For this review, use the dimensioned drawing (mm, ordinates from the lowest corner) and the shaded views. A direction names the side the tool comes from. Give positions to 0.01 mm unless a question says otherwise; leave off trailing zeros. Write each loop counter-clockwise with the first axis right and the second up, starting at its lowest first coordinate (ties: lowest second). Pieces come first, ordered by that corner, then holes. Notation, with made-up numbers: M 8,-21.5 L 39,-21.5 A33 cw 39,10.5 Z; hole C 46,74.25 d6. An arc over 180 degrees is marked long. One line per item, written item: value. Start each with the question number.
Item 1: Consider section C-C, the plane y = 2.25. Write out the cut boundary in (x, z), and give its area (3 significant figures).
Item 2: To check wall thickness, follow probe 1 along X at (y, z) = (2.75, 12); probe 2 along Z at (x, y) = (12.34, 1.75); probe 3 along Z at (x, y) = (21, 2.5). State the ranges of each line that lie inside material, in increasing order.
Item 3: Consider section B-B, the plane z = 12.34. Write out the cut boundary in (x, y), and give its area (3 significant figures).
Item 4: Mouldability with a two-part tool opening along X and no side actions: class the marked faces 3, 4 and 5 as released by +X, released by -X, zero draft, split by the parting line, or undercut.
Item 5: Consider section A-A, the plane x = 12.34. Write out the cut boundary in (y, z), and give its area (3 significant figures).
Item 6: Tool access review of the marked faces 1 and 2: name each direction out of +Z, -Z, +X, -X, +Y, -Y from which nothing blocks a thin tool from reaching the whole face with its end or side.
Item 7: Consider section D-D, the plane y = 8.25. Write out the cut boundary in (x, z).
Item 8: Clearance check with flat-ended pins moving along their axes: pin 1 Ø11 at (x, z) = (11.5, 12) entering from -Y; pin 2 Ø4 at (y, z) = (6.5, 15) entering from -X; pin 3 Ø2 at (x, z) = (5, 7) entering from -Y. State where each tip first meets the part, or that it passes through.
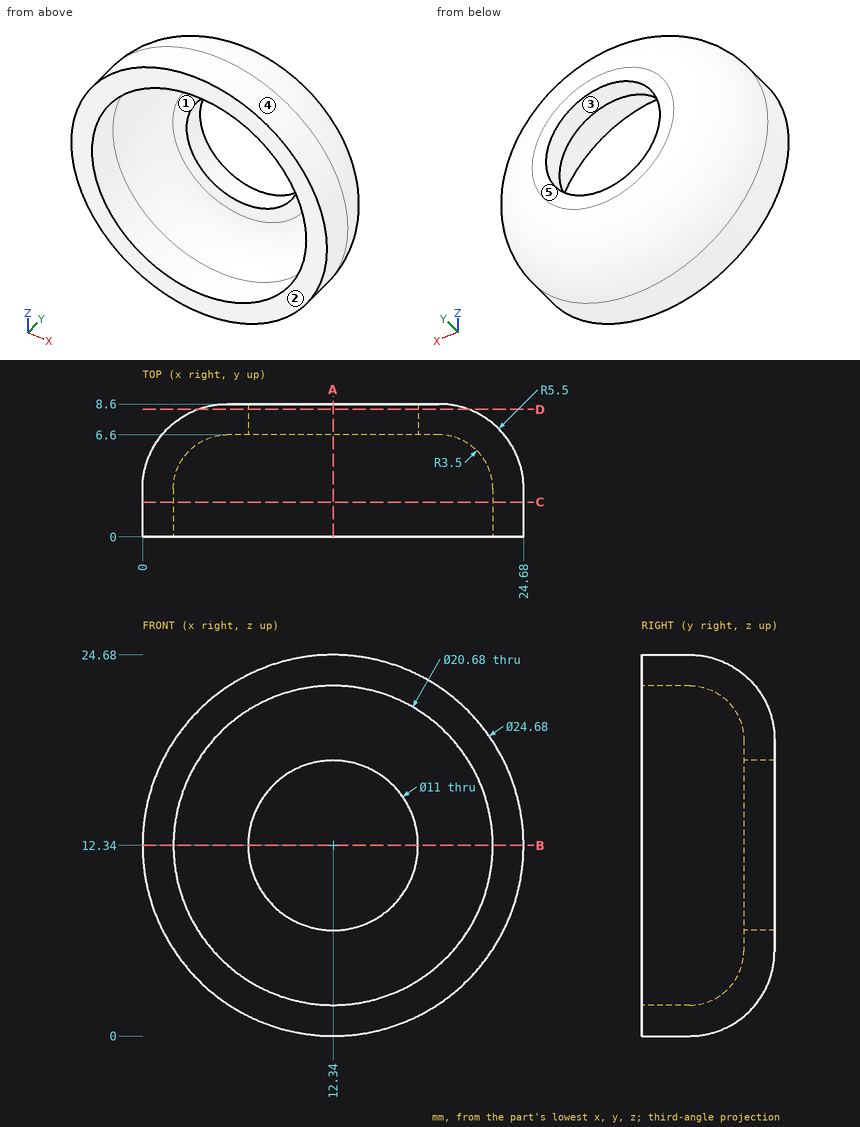
Model answer:
1. outline: C 12.34,12.34 d24.68; hole C 12.34,12.34 d20.68
1. area: 143 mm2
2. probe 1: x = 0 to 2.01, 22.67 to 24.68
2. probe 2: z = 0 to 2, 22.68 to 24.68
2. probe 3: z = 3.55 to 6.69, 17.99 to 21.13
3. outline: M 0,0 L 2,0 L 2,3.1 A3.5 cw 5.5,6.6 L 6.84,6.6 L 6.84,8.6 L 5.5,8.6 A5.5 ccw 0,3.1 Z; M 17.84,6.6 L 19.18,6.6 A3.5 cw 22.68,3.1 L 22.68,0 L 24.68,0 L 24.68,3.1 A5.5 ccw 19.18,8.6 L 17.84,8.6 Z
3. area: 46.0 mm2
4. face 3: undercut
4. face 4: split by the parting line
4. face 5: zero draft
5. outline: M 0,0 L 3.1,0 A5.5 ccw 8.6,5.5 L 8.6,6.84 L 6.6,6.84 L 6.6,5.5 A3.5 cw 3.1,2 L 0,2 Z; M 0,22.68 L 3.1,22.68 A3.5 cw 6.6,19.18 L 6.6,17.84 L 8.6,17.84 L 8.6,19.18 A5.5 ccw 3.1,24.68 L 0,24.68 Z
5. area: 46.0 mm2
6. face 1: -Y
6. face 2: +Z, -Z, +X, -X, -Y
7. outline: C 12.34,12.34 d17.54; hole C 12.34,12.34 d11
8. pin 1: stops at y = 6.6
8. pin 2: stops at x = 0.37
8. pin 3: stops at y = 4.43
